The listing builds one solid part. Answer for the finished solid, in the listing's coordinates (mm). Round coordinates to 2 decimals unless told otherwise and drop trailing zeros. Loops run counter-clockwise (first coordinate to the right, second up) from the corner with the lowest first, then second, coordinate; pieces in that order, holes last. Notation, with made-up numbers: M 77.25,21.5 L 99.25,21.5 A12 cw 99.25,31.5 Z; hole C 27,45 d5. An arc over 180 degrees is marked long. Answer as a JSON object with one key per item and string values.
Autodesk Inventor part; units mm, degrees
ref_plane "YZ Plane" through (0, 0, 0) normal (1, 0, 0) x (0, 1, 0)
ref_plane "XZ Plane" through (0, 0, 0) normal (0, 1, 0) x (-1, 0, 0)
ref_plane "XY Plane" through (0, 0, 0) normal (0, 0, 1) x (1, 0, 0)
sketch "Sketch1" plane through (0, 0, 0) normal (0, 0, 1) x (1, 0, 0)
  line L0 (-43.18, -27.305) -> (43.18, -27.305)
  line L1 (43.18, -27.305) -> (43.18, 27.305)
  line L2 (43.18, 27.305) -> (-43.18, 27.305)
  line L3 (-43.18, 27.305) -> (-43.18, -27.305)
  line L4 (-43.18, -27.305) -> (43.18, 27.305) construction
  line L5 (43.18, -27.305) -> (-43.18, 27.305) construction
  circle A0 centre (-40.64, 24.765) radius 1.5
  line L6 (-43.18, 0) -> (43.18, 0) construction
  line L7 (0, 27.305) -> (0, -27.305) construction
  circle A1 centre (-40.64, -24.765) radius 1.5
  circle A2 centre (40.64, 24.765) radius 1.5
  circle A3 centre (40.64, -24.765) radius 1.5
  point P0 (0, 0)
  dimension "d2" = 86.36
  dimension "d4" = 54.61
  dimension "d6" = 3
  dimension "d21" = 2.54
  dimension "d22" = 2.54
extrude "Extrusion1" add sketch "Sketch1" along normal blind 1
properties part number "Parallella" material "PCB(1)"
Item 1: The part is cut by section A-A (x = 40.64). Give the vertices of the cut face in (y, z) (3 decimals).
Values follow:
{"outline": "M -27.305,0 L -26.265,0 L -26.265,1 L -27.305,1 Z; M -23.265,0 L 23.265,0 L 23.265,1 L -23.265,1 Z; M 26.265,0 L 27.305,0 L 27.305,1 L 26.265,1 Z"}
Item 2: Determine the mould class of faces 1 (the face through (39.14, -24.83, 0.49)), 2 (the face through (-1, 0, 0)) for opening direction X: released by +X, released by -X, zero draft, split by the parting line, or undercut.
Values follow:
{"face 1": "undercut", "face 2": "zero draft"}
Item 3: Straight lines are drawn through the part: line 1 (Y direction, x = -40.64, z = 0.65) (3 decimals); line 2 (Y direction, x = 39.5, z = 0.05) (3 decimals); line 3 (X direction, y = 24.5, z = 0.95). For each, find the intervals that lie inside material, in ascending order.
Values follow:
{"line 1": "-27.305 to -26.265, -23.265 to 23.265, 26.265 to 27.305", "line 2": "-27.305 to -25.74, -23.79 to 23.79, 25.74 to 27.305", "line 3": "-43.18 to -42.12, -39.16 to 39.16, 42.12 to 43.18"}
